```python
from build123d import *

# Parameters (mm, degrees)
F0_W     = 209.55
F0_H     = 52.3875
F1_DEPTH = 57.15
F3_DEPTH = 76.2
F5_DEPTH = 76.2
F7_DEPTH = 72.644
F9_DEPTH = 19.304


with BuildPart() as f1:
    # F0 (on Front) → F1 (new body)
    with BuildSketch(Plane.XZ):
        with Locations((104.775, 26.19375)):
            Rectangle(F0_W, F0_H)
    extrude(amount=F1_DEPTH)

    # F2 (on face) → F3 (cut)
    with BuildSketch(Plane.XY.offset(52.3875)):
        Polygon((209.55, -57.15), (209.55, -28.575), (0, -57.15), align=None)
    extrude(amount=-F3_DEPTH, mode=Mode.SUBTRACT)

    # F4 (on face) → F5 (cut)
    with BuildSketch(Plane.XY.offset(52.3875)):
        Polygon((0, 0), (209.55, -28.575), (209.55, 0), align=None)
    extrude(amount=-F5_DEPTH, mode=Mode.SUBTRACT)

    # F6 (on face) → F7 (cut)
    with BuildSketch(Plane(origin=(7.650913, -56.106694, 0), x_dir=(0.99083, 0.135113, 0), z_dir=(0.135113, -0.99083, 0))):
        Polygon((-7.72172, 26.19375), (203.767602, 52.3875), (-7.72172, 52.3875), align=None)
    extrude(amount=-F7_DEPTH, mode=Mode.SUBTRACT)

    # F8 (on face) → F9 (cut)
    with BuildSketch(Plane(origin=(7.650913, -56.106694, 0), x_dir=(0.99083, 0.135113, 0), z_dir=(0.135113, -0.99083, 0))):
        Polygon((203.767602, 52.3875), (-7.72172, 26.19375), (-7.72172, 0), (203.767602, 0), align=None)
        Polygon((-7.72172, 0), (-7.72172, 26.19375), (-25.226625, 0), align=None)
    extrude(amount=F9_DEPTH, mode=Mode.SUBTRACT)


solid = f1.part
```
Design review of the part built by this model. Coordinates are the model's own, in mm. Coordinates: 2 decimals unless noted, no trailing zeros. Loops run counter-clockwise (first coordinate to the right, second up) from the corner with the lowest first, then second, coordinate; pieces in that order, holes last. Notation, with made-up numbers: M 24.25,32 L 48.25,32 A21 cw 48.25,42 Z; hole C 84.5,83 d11. An arc over 180 degrees is marked long. One line per question, with ' | ' between items.
(1) We need section A-A (z = 23). Give the boundary of the cut face in (x, y) (3 decimals).
Filled in:
outline: M 0,-57.15 L 5.917,-56.343 L 209.55,-28.575 L 0,0 Z
(2) We need section C-C (z = 33.5). Give the boundary of the cut face in (x, y) (3 decimals), and give its area (3 significant figures).
Filled in:
outline: M 52.724,-7.19 L 58.45,-49.18 L 209.55,-28.575 Z | area: 3,230 mm^2
(3) We need section B-B (y = -47.5). Give the boundary of the cut face in (x, z).
Filled in:
outline: M 0,0 L 70.77,0 L 70.77,35.04 L 0,26.36 Z
(4) Wall thickness on probe 1 along Y at (x, z) = (77, 27.5); probe 2 along Y at (x, z) = (183, 9); probe 3 along Z at (x, y) = (100.5, -23.5): over which ranges is each line inside the solid? List them lowest first.
Filled in:
probe 1: y = -46.65 to -10.5 | probe 2: y = -32.2 to -24.95 | probe 3: z = 0 to 39.09
(5) For pin 1 Ø4 at (x, z) = (174.5, 26) entering from -Y; pin 2 Ø6 at (x, z) = (122, 21) entering from +Y; pin 3 Ø8 at (x, y) = (128.5, -16) entering from +Z, all flat-tipped, find the tip position at first contact; note any pin that passes through.
Filled in:
pin 1: stops at y = -33.63 | pin 2: stops at y = -16.23 | pin 3: stops at z = 43.04
